Could you check a few things on this model? Use its own coordinates, in mm. Give positions to 0.01 mm unless a question says otherwise; leave off trailing zeros. Order: outer loops, then holes, each group sorted by start corner. A loop starts at its lowest first (then second) coordinate and runs counter-clockwise, first axis right, second up. Notation, with made-up numbers: (47.25, 84.25) -> (82.25, 84.25) arc R14 ccw to (82.25, 99.25) -> close; hole circle Ø2 at (60, -19.75). An arc over 180 degrees is marked (long way). Answer as CSV lines item,"result". Start each with the question number.
(1) We'd pull the mould along Z, two halves only. Please class faces 1 (the face through (154, 62, 3.175)), 2 (the face through (154, 62, 0)): released by +Z, released by -Z, zero draft, split by the parting line, or undercut.
(2) I want a section at B-B (x = 113.5). Please give me the cut outline in (y, z) (3 decimals).
(3) I want a section at A-A (y = 32.5). Please give me the cut outline in (x, z) (3 decimals).
(4) I want a section at C-C (z = 1.6). Give the number of separate pieces and of enclosed holes in the cut face, plus the area to 3 significant figures.
(5) Will these pins go through, and if not, where does the flat tip stop? pin 1 Ø1.5 at (y, z) = (32, 1) entering from +X (3 decimals); pin 2 Ø1 at (x, z) = (268.5, 1.5) entering from +Y.
(6) I need wall thicknesses on L1, parallel to X at y = 117, z = 1.85 (3 decimals); L2, parallel to X at y = 76.5, z = 2.45 (3 decimals); L3, parallel to Y at x = 177, z = 1.45. Which ranges of each line are inside material? Lowest first, please.
```python
from build123d import *

# Parameters (mm, degrees)
SKETCH1_R           = 1.5
SKETCH1_W           = 3.175
SKETCH1_H           = 24.635
BOSS_EXTRUDE1_DEPTH = 3.175


with BuildPart() as part:
    # Sketch1 → Boss-Extrude1 (new body)
    with BuildSketch(Plane.XY):
        Polygon((0, 0), (313, 0), (313, 24.635), (309.825, 24.635), (309.825, 49.27), (313, 49.27), (313, 73.905), (309.825, 73.905), (309.825, 98.54), (313, 98.54), (313, 123.175), (278.222222222, 123.175), (278.222222222, 120), (243.444444444, 120), (243.444444444, 123.175), (208.666666667, 123.175), (208.666666667, 120), (173.888888889, 120), (173.888888889, 123.175), (139.111111111, 123.175), (139.111111111, 120), (104.333333333, 120), (104.333333333, 123.175), (69.555555556, 123.175), (69.555555556, 120), (34.777777778, 120), (34.777777778, 123.175), (0, 123.175), (0, 98.54), (3.175, 98.54), (3.175, 73.905), (0, 73.905), (0, 49.27), (3.175, 49.27), (3.175, 24.635), (0, 24.635), align=None)
        with Locations((6.175, 117)):
            Circle(SKETCH1_R, mode=Mode.SUBTRACT)
        with Locations((108.920833333, 117)):
            Circle(SKETCH1_R, mode=Mode.SUBTRACT)
        with Locations(Location((108.920833333, 6.175, 0), (0, 0, 180))):
            Circle(SKETCH1_R, mode=Mode.SUBTRACT)
        with Locations(Location((6.175, 6.175, 0), (0, 0, 180))):
            Circle(SKETCH1_R, mode=Mode.SUBTRACT)
        with Locations((306.825, 6.175)):
            Circle(SKETCH1_R, mode=Mode.SUBTRACT)
        with Locations((204.079166667, 6.175)):
            Circle(SKETCH1_R, mode=Mode.SUBTRACT)
        with Locations(Location((204.079166667, 117, 0), (0, 0, 180))):
            Circle(SKETCH1_R, mode=Mode.SUBTRACT)
        with Locations(Location((306.825, 117, 0), (0, 0, 180))):
            Circle(SKETCH1_R, mode=Mode.SUBTRACT)
        with Locations((104.333333333, 86.2225)):
            Rectangle(SKETCH1_W, SKETCH1_H, mode=Mode.SUBTRACT)
        with Locations((104.333333333, 36.9525)):
            Rectangle(SKETCH1_W, SKETCH1_H, mode=Mode.SUBTRACT)
        with Locations((208.666666667, 86.2225)):
            Rectangle(SKETCH1_W, SKETCH1_H, mode=Mode.SUBTRACT)
        with Locations((208.666666667, 36.9525)):
            Rectangle(SKETCH1_W, SKETCH1_H, mode=Mode.SUBTRACT)
    extrude(amount=BOSS_EXTRUDE1_DEPTH)


solid = part.part
```
Final values:
1,face 1,"released by +Z"
1,face 2,"released by -Z"
2,outline,"(0, 0) -> (120, 0) -> (120, 3.175) -> (0, 3.175) -> close"
3,outline,"(3.175, 0) -> (102.746, 0) -> (102.746, 3.175) -> (3.175, 3.175) -> close; (105.921, 0) -> (207.079, 0) -> (207.079, 3.175) -> (105.921, 3.175) -> close; (210.254, 0) -> (309.825, 0) -> (309.825, 3.175) -> (210.254, 3.175) -> close"
4,separate pieces,"1"
4,enclosed holes,"12"
4,area,"37,400 mm²"
5,pin 1,"x = 309.825"
5,pin 2,"y = 120"
6,L1,"0 to 4.675, 7.675 to 107.421, 110.421 to 202.579, 205.579 to 305.325, 308.325 to 313"
6,L2,"3.175 to 102.746, 105.921 to 207.079, 210.254 to 309.825"
6,L3,"0 to 120"
